```python
from build123d import *

# Parameters (mm, degrees)
F0_W     = 118.4879094362
F0_H     = 85.4637138546
F1_DEPTH = 50
F2_SIZE  = 49.99999


# Not quite as in the source:
# - a fillet or chamfer is up to 0.001 mm smaller than in the source, because OpenCascade refuses the exact size


with BuildPart() as f1:
    # F0 (on Top) → F1 (new body)
    with BuildSketch(Plane.XY):
        with Locations((0.7258094847, -1.0887105018)):
            Rectangle(F0_W, F0_H)
    extrude(amount=F1_DEPTH)

    # F2 (size 50 in the source; OpenCascade refuses exactly that, so slightly less here)
    f2_edges = [f1.edges().sort_by_distance(p)[0] for p in [
        (0.725809, -43.820567, 50),
    ]]
    chamfer(f2_edges, length=F2_SIZE)


solid = f1.part
```
Design review of the part built by this model. Coordinates are the model's own, in mm. Coordinates: 2 decimals unless noted, no trailing zeros. Order: outer loops, then holes, each group sorted by start corner. A loop starts at its lowest first (then second) coordinate and runs counter-clockwise, first axis right, second up. Notation, with made-up numbers: M 56.5,10.5 L 107.5,10.5 A19 ccw 107.5,17.5 Z; hole C 36,7 d1. An arc over 180 degrees is marked long. Answer as a JSON object with one key per item and string values. Group by question number.
1) Wall thickness on L1, parallel to Z at x = 6, y = -39.5; L2, parallel to Y at x = 43.5, z = 42; L3, parallel to Y at x = -15.5, z = 26: over which ranges is each line inside the solid? List them lowest first.
2) For pin 1 (6 mm diameter, centred on x = -33, y = -32.5, fed in from +Z); pin 2 (6 mm diameter, centred on x = 22, z = 25, fed in from -Y); pin 3 (6 mm diameter, centred on x = 37.5, z = 26.5, fed in from -Y), all flat-tipped, find the tip position at first contact; note any pin that passes through.
3) Add section C-C, the plane z = 38. Write out the cut boundary in (x, y).
4) Add section B-B, the plane y = -35.5. Write out the cut boundary in (x, z), then the cut area to 3 significant figures.
Computed values:
{
 "1": {"L1": "z = 0 to 4.32", "L2": "y = -1.82 to 41.64", "L3": "y = -17.82 to 41.64"},
 "2": {"pin 1": "stops at z = 14.32", "pin 2": "stops at y = -21.82", "pin 3": "stops at y = -20.32"},
 "3": {"outline": "M -58.52,-5.82 L 59.97,-5.82 L 59.97,41.64 L -58.52,41.64 Z"},
 "4": {"outline": "M -58.52,0 L 59.97,0 L 59.97,8.32 L -58.52,8.32 Z", "area": "986 mm^2"}
}
